from build123d import *

# Parameters (mm, degrees)
BOSS_EXTRUDE1_DEPTH = 62
SKETCH2_W           = 10
SKETCH2_H           = 60
CUT_EXTRUDE1_DEPTH  = 85
SKETCH12_W          = 44
SKETCH12_H          = 51.120506265
CUT_EXTRUDE11_DEPTH = 30
SKETCH17_R          = 2.75
SKETCH17_R_2        = 32.5
CUT_EXTRUDE14_DEPTH = 6
CUT_EXTRUDE17_DEPTH = 10
CUT_EXTRUDE18_DEPTH = 6
SKETCH24_W          = 44
SKETCH24_H          = 8.565563784
CUT_EXTRUDE19_DEPTH = 31.0000001
BOSS_EXTRUDE2_DEPTH = 12.5
BOSS_EXTRUDE3_DEPTH = 5
CUT_EXTRUDE20_START = -0.6
CUT_EXTRUDE20_DEPTH = 3.4
SKETCH29_R          = 2.75
CUT_EXTRUDE21_DEPTH = 6
SKETCH33_R          = 2.75
BOSS_EXTRUDE5_DEPTH = 0.4


with BuildPart() as part:
    # Sketch1 → Boss-Extrude1 (new body)
    with BuildSketch(Plane.XY):
        with BuildLine():
            Line((-42, 0), (42, 0))
            Line((42, 0), (42, 5))
            Line((42, 5), (27, 5))
            Line((27, 5), (27, 65))
            Line((27, 65), (4, 65))
            ThreePointArc((4, 65), (0, 61), (-4, 65))
            Line((-4, 65), (-27, 65))
            Line((-27, 65), (-27, 5))
            Line((-27, 5), (-42, 5))
            Line((-42, 5), (-42, 0))
        make_face()
        with BuildLine():
            Line((-11.5, 37), (-11.5, 33))
            ThreePointArc((-11.5, 33), (0, 21.5), (11.5, 33))
            Line((11.5, 33), (11.5, 37))
            ThreePointArc((11.5, 37), (0, 48.5), (-11.5, 37))
        make_face(mode=Mode.SUBTRACT)
    extrude(amount=BOSS_EXTRUDE1_DEPTH)

    # Sketch2 → Cut-Extrude1 (cut, through all)
    with BuildSketch(Plane.ZY.offset(42)):
        with Locations((5, 35)):
            Rectangle(SKETCH2_W, SKETCH2_H)
        with BuildLine():
            Line((62, 5), (62, 65))
            Line((62, 65), (15.5, 65))
            ThreePointArc((15.5, 65), (29.081460906, 27.506882202), (62, 5))
        make_face()
    extrude(amount=-CUT_EXTRUDE1_DEPTH, mode=Mode.SUBTRACT)

    # Sketch12 → Cut-Extrude11 (cut)
    with BuildSketch(Plane(origin=(0, 5, 0), x_dir=(1, 0, 0), z_dir=(0, 1, 0))):
        with Locations((0, -41.060253133)):
            Rectangle(SKETCH12_W, SKETCH12_H)
    extrude(amount=CUT_EXTRUDE11_DEPTH, mode=Mode.SUBTRACT)

    # Sketch17 → Cut-Extrude14 (cut, through all)
    with BuildSketch(Plane(origin=(0, 5, 0), x_dir=(1, 0, 0), z_dir=(0, 1, 0))):
        with Locations(Location((-36, -6, 0), (0, 0, 180))):  # turned: the seam where the file's is
            Circle(SKETCH17_R)
        with Locations(Location((36, -6, 0), (0, 0, 180))):  # turned: the seam where the file's is
            Circle(SKETCH17_R)
        with Locations(Location((36, -56, 0), (0, 0, 180))):  # turned: the seam where the file's is
            Circle(SKETCH17_R)
        with Locations(Location((-36, -56, 0), (0, 0, 180))):  # turned: the seam where the file's is
            Circle(SKETCH17_R)
        with Locations((65.278831944, -31)):
            Circle(SKETCH17_R_2)
        with Locations((-65.278831944, -31)):
            Circle(SKETCH17_R_2)
    extrude(amount=-CUT_EXTRUDE14_DEPTH, mode=Mode.SUBTRACT)

    # Sketch20 → Cut-Extrude17 (cut)
    with BuildSketch(Plane.XY.offset(15.5)):
        with BuildLine():
            Line((-17.5, 52.5), (-17.5, 48.5))
            ThreePointArc((-17.5, 48.5), (-15.5, 46.5), (-13.5, 48.5))
            Line((-13.5, 48.5), (-13.5, 52.5))
            ThreePointArc((-13.5, 52.5), (-15.5, 54.5), (-17.5, 52.5))
        make_face()
        with BuildLine():
            Line((13.5, 52.5), (13.5, 48.5))
            ThreePointArc((13.5, 48.5), (15.5, 46.5), (17.5, 48.5))
            Line((17.5, 48.5), (17.5, 52.5))
            ThreePointArc((17.5, 52.5), (15.5, 54.5), (13.5, 52.5))
        make_face()
        with BuildLine():
            Line((-17.5, 21.5), (-17.5, 17.5))
            ThreePointArc((-17.5, 17.5), (-15.5, 15.5), (-13.5, 17.5))
            Line((-13.5, 17.5), (-13.5, 21.5))
            ThreePointArc((-13.5, 21.5), (-15.5, 23.5), (-17.5, 21.5))
        make_face()
        with BuildLine():
            Line((13.5, 17.5), (13.5, 21.5))
            ThreePointArc((13.5, 21.5), (15.5, 23.5), (17.5, 21.5))
            Line((17.5, 21.5), (17.5, 17.5))
            ThreePointArc((17.5, 17.5), (15.5, 15.5), (13.5, 17.5))
        make_face()
    extrude(amount=-CUT_EXTRUDE17_DEPTH, mode=Mode.SUBTRACT)

    # Sketch21 → Cut-Extrude18 (cut, through all)
    with BuildSketch(Plane(origin=(0, 5, 0), x_dir=(1, 0, 0), z_dir=(0, 1, 0))):
        with BuildLine():
            Line((-12, -20.5), (12, -20.5))
            ThreePointArc((12, -20.5), (15.535533906, -21.964466094), (17, -25.5))
            Line((17, -25.5), (17, -49))
            ThreePointArc((17, -49), (15.535533906, -52.535533906), (12, -54))
            Line((12, -54), (-12, -54))
            ThreePointArc((-12, -54), (-15.535533906, -52.535533906), (-17, -49))
            Line((-17, -49), (-17, -25.5))
            ThreePointArc((-17, -25.5), (-15.535533906, -21.964466094), (-12, -20.5))
        make_face()
    extrude(amount=-CUT_EXTRUDE18_DEPTH, mode=Mode.SUBTRACT)

    # Sketch24 → Cut-Extrude19 (cut, through all)
    with BuildSketch(Plane.XZ.offset(-35)):
        with Locations((0, 19.782781892)):
            Rectangle(SKETCH24_W, SKETCH24_H)
    extrude(amount=-CUT_EXTRUDE19_DEPTH, mode=Mode.SUBTRACT)

    # Sketch25 → Boss-Extrude2 (add)
    with BuildSketch(Plane(origin=(0, 0, 10), x_dir=(-1, 0, 0), z_dir=(0, 0, -1))):
        with BuildLine():
            Line((-27, 65), (-4, 65))
            ThreePointArc((-4, 65), (0, 61), (4, 65))
            Line((4, 65), (27, 65))
            Line((27, 65), (27, 56))
            Line((27, 56), (-27, 56))
            Line((-27, 56), (-27, 65))
        make_face()
    extrude(amount=BOSS_EXTRUDE2_DEPTH)

    # Sketch27 → Boss-Extrude3 (add)
    with BuildSketch(Plane.ZY.offset(27)):
        with BuildLine():
            Line((-2.5, 56), (10, 56))
            Line((10, 56), (10, 5))
            Line((10, 5), (0, 5))
            ThreePointArc((0, 5), (6.947455101, 30.901836034), (-2.5, 56))
        make_face()
    boss_extrude3 = extrude(amount=-BOSS_EXTRUDE3_DEPTH)

    # Mirror1: Boss-Extrude3 across plane
    add(boss_extrude3.mirror(Plane(origin=(0, 0, 0), x_dir=(0, 0, 1), z_dir=(1, 0, 0))))

    # Sketch28 → Cut-Extrude20 (cut)
    with BuildSketch(Plane.XZ.offset(-56).offset(CUT_EXTRUDE20_START)):
        Polygon((-5.092522712, 5.5), (-7.546261356, 9.75), (-12.453738644, 9.75), (-14.907477288, 5.5), (-12.453738644, 1.25), (-7.546261356, 1.25), align=None)
        Polygon((5.092522712, 5.5), (7.546261356, 1.25), (12.453738644, 1.25), (14.907477288, 5.5), (12.453738644, 9.75), (7.546261356, 9.75), align=None)
    extrude(amount=-CUT_EXTRUDE20_DEPTH, mode=Mode.SUBTRACT)

    # Sketch29 → Cut-Extrude21 (cut)
    with BuildSketch(Plane(origin=(0, 65, 0), x_dir=(1, 0, 0), z_dir=(0, 1, 0))):
        with Locations(Location((-10, -5.5, 0), (0, 0, 270))):  # turned: the seam where the file's is
            Circle(SKETCH29_R)
        with Locations(Location((10, -5.5, 0), (0, 0, 270))):  # turned: the seam where the file's is
            Circle(SKETCH29_R)
    extrude(amount=-CUT_EXTRUDE21_DEPTH, mode=Mode.SUBTRACT)

    # Sketch33 → Boss-Extrude5 (add)
    with BuildSketch(Plane.XZ.offset(-60)):
        with Locations(Location((10, 5.5, 0), (0, 0, 90))):  # turned: the seam where the file's is
            Circle(SKETCH33_R)
        with Locations(Location((-10, 5.5, 0), (0, 0, 90))):  # turned: the seam where the file's is
            Circle(SKETCH33_R)
    extrude(amount=-BOSS_EXTRUDE5_DEPTH)


solid = part.part
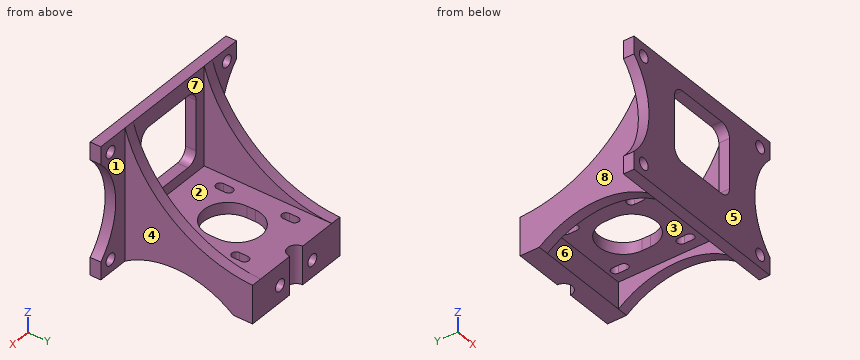
The model under review builds one solid part; all positions refer to its coordinate system, in mm. Face numbers are marked on the shaded views. A direction names the side the tool comes from. Round coordinates to 2 decimals unless told otherwise and drop trailing zeros. Write each loop counter-clockwise with the first axis right and the second up, starting at its lowest first coordinate (ties: lowest second). Pieces come first, ordered by that corner, then holes. Notation, with made-up numbers: M -29,57 L 14,57 A27 cw 14,84 Z; hole C 89,-0.75 d3. An arc over 180 degrees is marked long. Answer as CSV lines item,"result". Start each with the question number.
Q1. Clearance check with flat-ended pins moving along their axes: P1, Ø1, axis at x = 14.5, z = 21, coming from the +Y side; P2, Ø2, axis at y = 49.5, z = 12, coming from the +X side; P3, Ø1.2, axis at y = 20.5, z = 12.5, coming from the -X side; P4, Ø23, axis at y = 34, z = 49.5, coming from the -X side. State where each tip first meets the part, or that it passes through.
Q2. Tool access review of the marked faces 4, 5, 6, 7 and 8: name each direction out of +Z, -Z, +X, -X, +Y, -Y from which nothing blocks a thin tool from reaching the whole face with its end or side.
Q3. The part is to be moulded in two halves that separate along Y. For the marked faces 1, 2 and 3, say which applies: +Y half, -Y half, draft (parallel to the pull), parting line (faces both ways), or undercut.
Q4. Consider section C-C, the plane y = 51. Give the boundary of the cut face in (x, z), then the cut area to 3 significant figures.
Q5. Wall thickness on line 1 along Z through (x, y) = (36, 3.35); line 2 along X through (y, z) = (13, 30); line 3 along Z through (x, y) = (-10, 63): over which ranges is each line inside the solid? List them lowest first.
Q6. Consider section D-D, the plane x = 0. Give the boundary of the cut face in (y, z), then the cut area to 4 significant figures.
Q7. Consider section A-A, the plane x = -10. Give the boundary of the cut face in (y, z).
Q8. Consider section B-B, the plane z = 56. Give the boundary of the cut face in (x, y).
Result set:
1,P1,"stops at y = 5"
1,P2,"stops at x = 27"
1,P3,"stops at x = -27"
1,P4,"passes through"
2,face 4,"+Z, -Z, +X, +Y"
2,face 5,"+Z, -Z, +X, -X, -Y"
2,face 6,"-Z"
2,face 7,"+Z, +Y"
2,face 8,"+Z, -Z, -X, +Y"
3,face 1,"+Y half"
3,face 2,"draft"
3,face 3,"undercut"
4,outline,"M -27,0.93 L -22,0.93 L -22,10 L -17.5,10 L -17.5,15.5 L -22,15.5 L -22,17.54 L -27,17.54 Z; M -13.5,10 L 13.5,10 L 13.5,15.5 L -13.5,15.5 Z; M 17.5,10 L 22,10 L 22,0.93 L 27,0.93 L 27,17.54 L 22,17.54 L 22,15.5 L 17.5,15.5 Z"
4,area,"364 mm²"
5,line 1,"z = 0 to 3.25, 8.75 to 16.89, 45.11 to 53.25, 58.75 to 62"
5,line 2,"x = -27 to -22, 22 to 27"
5,line 3,"z = -2.5 to 2.75, 8.25 to 15.5"
6,outline,"M 0,0 L 5,0 L 5,10 L 21.5,10 L 21.5,15.5 L 5,15.5 L 5,20.5 L 0,20.5 Z; M 0,54 L 5,54 L 5,62 L 0,62 Z; M 48.5,10 L 56,10 L 56,-2.5 L 61,-2.5 L 61,15.5 L 48.5,15.5 Z"
6,area,"364.5 mm²"
7,outline,"M 0,0 L 5,0 L 5,10 L 27.32,10 L 27.32,15.5 L 5,15.5 L 5,20.5 L 0,20.5 Z; M 0,54 L 5,54 L 5,62 L 0,62 Z; M 42.68,10 L 56,10 L 56,-2.5 L 65,-2.5 L 65,2.75 L 60.4,2.75 L 60.4,8.25 L 65,8.25 L 65,15.5 L 42.68,15.5 Z; hole M 56.6,1.25 L 60,1.25 L 60,9.75 L 56.6,9.75 Z"
8,outline,"M -42,0 L -38.75,0 L -38.75,5 L -42,5 Z; M -33.25,0 L 33.25,0 L 33.25,5 L 27,5 L 27,7.1 L 22,7.1 L 22,5 L -22,5 L -22,7.1 L -27,7.1 L -27,5 L -33.25,5 Z; M 38.75,0 L 42,0 L 42,5 L 38.75,5 Z"
